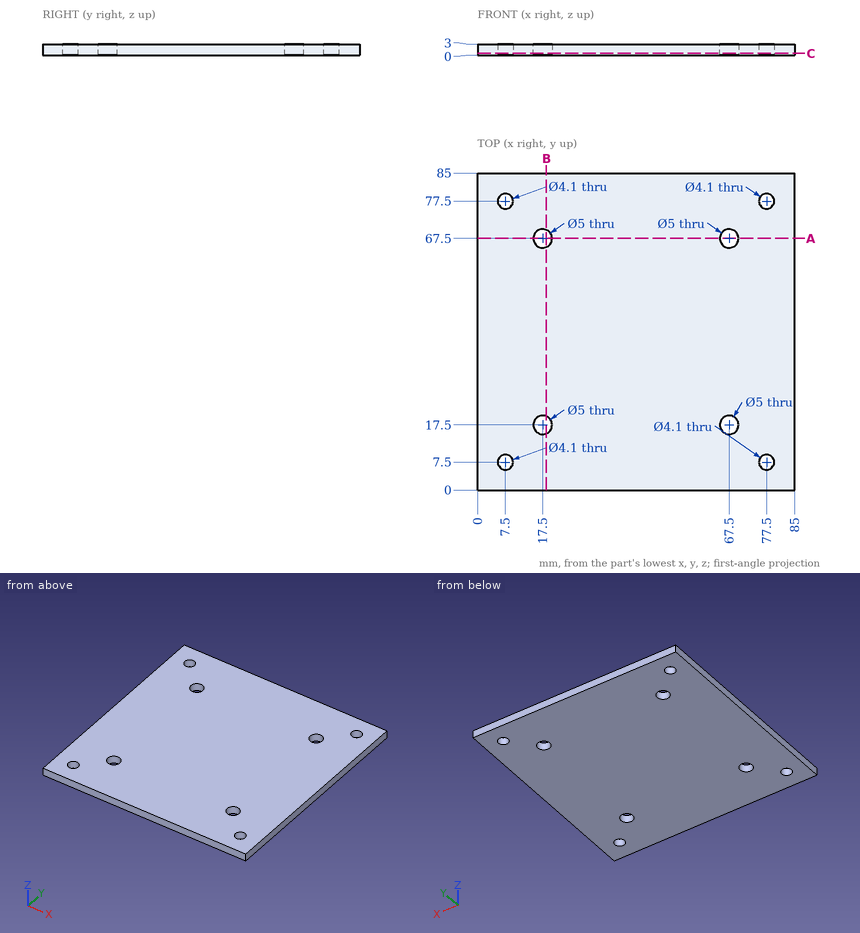
Job drawing, mm, ordinate dimensions from the low corner. One solid piece. Give positions to 0.01 mm unless a question says otherwise; leave off trailing zeros. Write each loop counter-clockwise with the first axis right and the second up, starting at its lowest first coordinate (ties: lowest second). Pieces come first, ordered by that corner, then holes. Notation, with made-up numbers: (-26, 89) - (32, 89) arc R21 ccw to (32, 118) - close; hole circle Ø10 at (5.25, -31). An arc over 180 degrees is marked (long way). Use one line per item in the form item = value. Start each with the question number.
1. Probe line 1 (Y direction, x = 17.5, z = 1.85); line 2 (X direction, y = 77.5, z = 1.7). List the from-to ranges inside material, lowest first. Write a range as [from, to].
2. Band-saw the part on C-C on z = 0.5. Count the separate pieces of the cut face and the enclosed holes in it, plus the area to 3 significant figures.
3. Band-saw the part on A-A on y = 67.5. Write the cut outline in (x, z).
4. Band-saw the part on B-B on x = 18.5. Write the cut outline in (y, z), plus the area to 3 significant figures.
Conclusion:
q1.line_1 = [0, 15], [20, 65], [70, 85]
q1.line_2 = [0, 5.45], [9.55, 75.45], [79.55, 85]
q2.separate_pieces = 1
q2.enclosed_holes = 8
q2.area = 7,090 mm²
q3.outline = (0, 0) - (15, 0) - (15, 3) - (0, 3) - close; (20, 0) - (65, 0) - (65, 3) - (20, 3) - close; (70, 0) - (85, 0) - (85, 3) - (70, 3) - close
q4.outline = (0, 0) - (15.21, 0) - (15.21, 3) - (0, 3) - close; (19.79, 0) - (65.21, 0) - (65.21, 3) - (19.79, 3) - close; (69.79, 0) - (85, 0) - (85, 3) - (69.79, 3) - close
q4.area = 228 mm²
